```python
from build123d import *

# Parameters (mm, degrees)
CYLINDER004_R     = 1
CYLINDER004_DEPTH = 10
CYLINDER005_R     = 1
CYLINDER005_DEPTH = 10
CYLINDER003_R     = 1
CYLINDER003_DEPTH = 10
CYLINDER002_R     = 1
CYLINDER002_DEPTH = 10
CYLINDER_R        = 3
CYLINDER_DEPTH    = 10
CYLINDER001_R     = 3
CYLINDER001_DEPTH = 10
BOX_W             = 44
BOX_H             = 44
BOX_DEPTH         = 6


with BuildPart() as cylinder004:
    # Cylinder004 → Cylinder004 (new body)
    with BuildSketch(Plane(origin=(19, 39, -2), x_dir=(1, 0, 0), z_dir=(0, 0, 1))):
        Circle(CYLINDER004_R)
    extrude(amount=CYLINDER004_DEPTH)


with BuildPart() as cylinder005:
    # Cylinder005 → Cylinder005 (new body)
    with BuildSketch(Plane(origin=(25, 39, -2), x_dir=(1, 0, 0), z_dir=(0, 0, 1))):
        Circle(CYLINDER005_R)
    extrude(amount=CYLINDER005_DEPTH)


with BuildPart() as cylinder003:
    # Cylinder003 → Cylinder003 (new body)
    with BuildSketch(Plane(origin=(25, 5, -2), x_dir=(1, 0, 0), z_dir=(0, 0, 1))):
        Circle(CYLINDER003_R)
    extrude(amount=CYLINDER003_DEPTH)


with BuildPart() as cylinder002:
    # Cylinder002 → Cylinder002 (new body)
    with BuildSketch(Plane(origin=(19, 5, -2), x_dir=(1, 0, 0), z_dir=(0, 0, 1))):
        Circle(CYLINDER002_R)
    extrude(amount=CYLINDER002_DEPTH)


with BuildPart() as cylinder:
    # Cylinder → Cylinder (new body)
    with BuildSketch(Plane(origin=(22, 5, 3), x_dir=(1, 0, 0), z_dir=(0, 0, 1))):
        Circle(CYLINDER_R)
    extrude(amount=CYLINDER_DEPTH)


with BuildPart() as cylinder001:
    # Cylinder001 → Cylinder001 (new body)
    with BuildSketch(Plane(origin=(22, 39, 3), x_dir=(1, 0, 0), z_dir=(0, 0, 1))):
        Circle(CYLINDER001_R)
    extrude(amount=CYLINDER001_DEPTH)


with BuildPart() as cut005:
    # Box → Box (new body)
    with BuildSketch(Plane.XY):
        with Locations((22, 22)):
            Rectangle(BOX_W, BOX_H)
    extrude(amount=BOX_DEPTH)

    # Cut: cut Cylinder001
    add(cylinder001.part, mode=Mode.SUBTRACT)

    # Cut001: cut Cylinder
    add(cylinder.part, mode=Mode.SUBTRACT)

    # Cut002: cut Cylinder002
    add(cylinder002.part, mode=Mode.SUBTRACT)

    # Cut003: cut Cylinder003
    add(cylinder003.part, mode=Mode.SUBTRACT)

    # Cut004: cut Cylinder005
    add(cylinder005.part, mode=Mode.SUBTRACT)

    # Cut005: cut Cylinder004
    add(cylinder004.part, mode=Mode.SUBTRACT)


solid = cut005.part
```
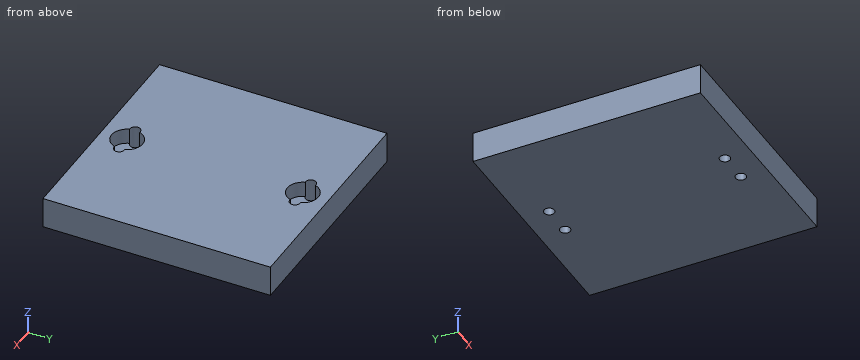
Source: CAD feature listing. Evaluate the final solid. Frame: model axes, mm. Round coordinates to 2 decimals unless told otherwise and drop trailing zeros. Loops run counter-clockwise (first coordinate to the right, second up) from the corner with the lowest first, then second, coordinate; pieces in that order, holes last. Notation, with made-up numbers: M 6.5,-37.75 L 18.5,-37.75 A35 ccw 18.5,-2.75 Z; hole C -19.75,3.25 d1. An arc over 180 degrees is marked long. Use a Markdown table: item, result. Add a question column.
1. Ray query, line 1 along Y through (x, z) = (19, 2.8); line 2 along X through (y, z) = (39, 1.9); line 3 along X through (y, z) = (39, 3.6). Return the intervals inside material, ascending. Write a range as [from, to].
2. Cut plane B-B, the plane z = 4.3. Output: boundary loops of the cut face in (x, y).
3. Cut plane A-A, the plane y = 39. Output: boundary loops of the cut face in (x, z), and give its area (3 significant figures).
4. Contact query for flat-ended pins moving along their axis: pin 1 (3 mm diameter, centred on x = 23, y = 38, fed in from +Z); pin 2 (1.6 mm diameter, centred on x = 25, y = 39, fed in from -Z). Output: stop coordinate, or through.
Solution:
| question | item | result |
|---|---|---|
| 1 | line 1 | y = [0, 4], [6, 38], [40, 44] |
| 1 | line 2 | x = [0, 18], [20, 24], [26, 44] |
| 1 | line 3 | x = [0, 18], [26, 44] |
| 2 | outline | M 0,0 L 44,0 L 44,44 L 0,44 Z; hole M 19.17,4.01 A3 ccw 24.83,4.01 A1 ccw long 24.83,5.99 A3 ccw 19.17,5.99 A1 ccw long Z; hole M 19.17,38.01 A3 ccw 24.83,38.01 A1 ccw long 24.83,39.99 A3 ccw 19.17,39.99 A1 ccw long Z |
| 3 | outline | M 0,0 L 18,0 L 18,6 L 0,6 Z; M 20,0 L 24,0 L 24,3 L 20,3 Z; M 26,0 L 44,0 L 44,6 L 26,6 Z |
| 3 | area | 228 mm2 |
| 4 | pin 1 | stops at z = 3 |
| 4 | pin 2 | passes through |
